Can you work these out from the model? Positions are in its coordinate system, mm. Face numbers are marked on the shaded views. Round coordinates to 2 decimals unless told otherwise and drop trailing zeros. Write each loop counter-clockwise with the first axis right and the second up, starting at its lowest first coordinate (ties: lowest second). Pieces come first, ordered by that corner, then holes. Notation, with made-up numbers: M 89,71.5 L 115,71.5 A15 cw 115,96.5 Z; hole C 49.25,62.5 d6. An arc over 180 degrees is marked long. Answer in a Markdown table with one row per item. Add a question column.
(1) Suppose I cut it at C-C, the plane x = -20. Write out the boundary of the cut face in (y, z).
(2) If I drill on probe 1 along X at (y, z) = (9.5, 25); probe 2 along Z at (x, y) = (-0.5, 0.5); probe 3 along X at (y, z) = (9.25, 24), over which ranges is the centre line in solid material (lowest first)?
(3) If we mould it in two halves opening along X, with no side actions, what happens to the marked faces 1, 2 and 3? For each: released by +X, released by -X, zero draft, split by the parting line, or undercut.
(4) Suppose I cut it at B-B, the plane z = -31.5. Write out the boundary of the cut face in (x, y).
(5) Suppose I cut it at A-A, the plane x = 0. Write out the boundary of the cut face in (y, z), then the cut area to 3 significant figures.
(6) Suppose I cut it at D-D, the plane y = 9. Count the separate pieces of the cut face and the enclosed holes in it, then the cut area to 3 significant figures.
(7) I'm going to push flat-ended pins straight in: pin 1 (5 mm diameter, centred on y = 1.5, z = -20.5, fed in from -X); pin 2 (1 mm diameter, centred on x = 5, y = 9.5, fed in from -Z); pin 3 (0.9 mm diameter, centred on x = 3.5, z = 16, fed in from +Y). Where does each tip first touch, or does it pass through?
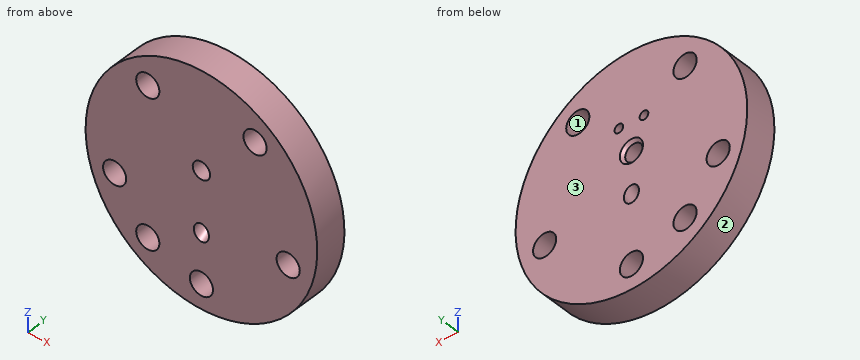
from build123d import *

# Parameters (mm, degrees)
SKETCH_1_R          = 40
SKETCH_1_R_2        = 4
EXTRUDE_1_DEPTH     = 11
SKETCH_3_R          = 3
CUT_EXTRUDE_1_DEPTH = 58.628118137
CHAMFER_1_SIZE      = 1
SKETCH_6_R          = 2.6
CUT_EXTRUDE_2_DEPTH = 10
SKETCH_7_R          = 1.5
CUT_EXTRUDE_3_DEPTH = 8


with BuildPart() as part:
    # Sketch 1 → Extrude 1 (new body)
    with BuildSketch(Plane(origin=(0, 0, 0), x_dir=(1, 0, 0), z_dir=(0, 1, 0))):
        with Locations(Location((0, 0, 0), (0, 0, 270))):
            Circle(SKETCH_1_R)
        with Locations(Location((0, 31.5, 0), (0, 0, 270))):
            Circle(SKETCH_1_R_2, mode=Mode.SUBTRACT)
        with Locations(Location((29.958280263, 9.734035323, 0), (0, 0, 270))):
            Circle(SKETCH_1_R_2, mode=Mode.SUBTRACT)
        with Locations(Location((18.515235447, -25.484035323, 0), (0, 0, 270))):
            Circle(SKETCH_1_R_2, mode=Mode.SUBTRACT)
        with Locations(Location((-18.515235447, -25.484035323, 0), (0, 0, 270))):
            Circle(SKETCH_1_R_2, mode=Mode.SUBTRACT)
        with Locations(Location((-29.958280263, 9.734035323, 0), (0, 0, 270))):
            Circle(SKETCH_1_R_2, mode=Mode.SUBTRACT)
        with Locations(Location((-18.515235447, 25.484035323, 0), (0, 0, 270))):
            Circle(SKETCH_1_R_2, mode=Mode.SUBTRACT)
    extrude(amount=EXTRUDE_1_DEPTH)

    # Sketch 3 → Cut-Extrude 1 (cut, through all)
    with BuildSketch(Plane(origin=(0, 11, 0), x_dir=(1, 0, 0), z_dir=(0, 1, 0))):
        with Locations(Location((0, -6.456029322, 0), (0, 0, 270))):
            Circle(SKETCH_3_R)
    extrude(amount=-CUT_EXTRUDE_1_DEPTH, mode=Mode.SUBTRACT)

    # Chamfer 1
    chamfer_1_edges = [part.edges().sort_by_distance(p)[0] for p in [
        (0, 11, 3.456029322),
    ]]
    chamfer(chamfer_1_edges, length=CHAMFER_1_SIZE)

    # Sketch 6 → Cut-Extrude 2 (cut, symmetric)
    with BuildSketch(Plane(origin=(0, 0, 0), x_dir=(1, 0, 0), z_dir=(0, 0.8660254037844398, 0.499999999999998))):
        with Locations(Location((0, 12.42820323, 0), (0, 0, 270))):
            Circle(SKETCH_6_R)
    extrude(amount=CUT_EXTRUDE_2_DEPTH, both=True, mode=Mode.SUBTRACT)

    # Sketch 7 → Cut-Extrude 3 (cut)
    with BuildSketch(Plane(origin=(0, 11, 0), x_dir=(1, 0, 0), z_dir=(0, 1, 0))):
        with Locations(Location((-4.335219005, -16.17925759, 0), (0, 0, 270))):
            Circle(SKETCH_7_R)
        with Locations(Location((4.335219005, -16.17925759, 0), (0, 0, 270))):
            Circle(SKETCH_7_R)
    extrude(amount=-CUT_EXTRUDE_3_DEPTH, mode=Mode.SUBTRACT)


solid = part.part
Calculated:
| question | item | result |
|---|---|---|
| 1 | outline | M 0,-34.64 L 11,-34.64 L 11,-29.2 L 0,-29.2 Z; M 0,-21.77 L 11,-21.77 L 11,21.77 L 0,21.77 Z; M 0,29.2 L 11,29.2 L 11,34.64 L 0,34.64 Z |
| 2 | probe 1 | -31.22 to -22.49, -14.54 to 14.54, 22.49 to 31.22 |
| 2 | probe 2 | -40 to -35.47, -27.53 to -17.01, -11.12 to 3.5, 9.41 to 40 |
| 2 | probe 3 | -32 to -22.23, -14.8 to 14.8, 22.23 to 32 |
| 3 | face 1 | undercut |
| 3 | face 2 | split by the parting line |
| 3 | face 3 | zero draft |
| 4 | outline | M -24.65,0 L -4,0 L -4,11 L -24.65,11 Z; M 4,0 L 24.65,0 L 24.65,11 L 4,11 Z |
| 5 | outline | M 0,-40 L 11,-40 L 11,-35.5 L 0,-35.5 Z; M 0,-27.5 L 11,-27.5 L 11,-11 L 0,-17.35 Z; M 0,-11.35 L 11,-5 L 11,2.46 L 10,3.46 L 0,3.46 Z; M 0,9.46 L 10,9.46 L 11,10.46 L 11,40 L 0,40 Z |
| 5 | area | 659 mm² |
| 6 | separate pieces | 1 |
| 6 | enclosed holes | 10 |
| 6 | area | 4,660 mm² |
| 7 | pin 1 | x = -35.72 |
| 7 | pin 2 | z = -39.75 |
| 7 | pin 3 | y = 3 |
